Read the model definition and answer for the solid it produces. Units are mm, in the model's axes. Face numbers are marked on the shaded views. A direction names the side the tool comes from. Round coordinates to 2 decimals unless told otherwise and drop trailing zeros. Order: outer loops, then holes, each group sorted by start corner. A loop starts at its lowest first (then second) coordinate and runs counter-clockwise, first axis right, second up. Notation, with made-up numbers: (10.25, 32.25) - (17.25, 32.25) arc R8 ccw to (17.25, 37.25) - close; hole circle Ø7 at (-3, 83.25). An arc over 180 degrees is marked (long way). Answer as a JSON object with one key per item and string values. Group by question number.
Q1. The mould has two halves that part along Z. Classify the marked faces 1, 2, 3 and 4: pulls with the +Z half, pulls with the -Z half, needs draft (parallel to the pull), parting line crosses it, or undercut.
Q2. A tool of negligible diameter and unlimited length cuts with its end or side. For the marked faces 5, 6, 7 and 8, from which of +Z, -Z, +X, -X, +Y, -Y can it reach the whole face along a straight path? Write none if from no direction.
Q3. Consider line 1 (Z direction, x = 18.25, y = 0); line 2 (Z direction, x = 25.5, y = 13); line 3 (X direction, y = -1.5, z = 4.75). Determine where each line is inside the solid, lowest interval first.
Q4. A cutting plane is placed at D-D on z = 0. Determine the outline of the cut face in (x, y), and give its area (3 significant figures).
Q5. A cutting plane is placed at B-B on x = 16.75. Determine the outline of the cut face in (y, z), and give its area (3 significant figures).
Q6. A cutting plane is placed at C-C on y = 0. Determine the outline of the cut face in (x, z).
Q7. Given pin 1 Ø0.5 at (y, z) = (22, -4.5) entering from -X; pin 2 Ø1.1 at (y, z) = (23, -7) entering from +X; pin 3 Ø5 at (x, y) = (22, 23) entering from +Z; pin 4 Ø2.5 at (x, y) = (25, 12.5) entering from -Z, each flat-ended and moving along its own axis, determine where each tip first touches the part or whether it passes through.
Q8. A cutting plane is placed at A-A on y = 25. Determine the outline of the cut face in (x, z), and give its area (3 significant figures).
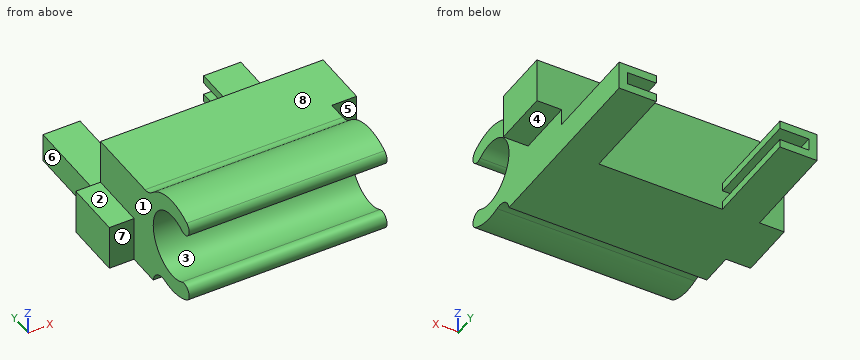
Autodesk Inventor part; units mm, degrees
ref_plane "YZ Plane" through (0, 0, 0) normal (1, 0, 0) x (0, 1, 0)
ref_plane "XZ Plane" through (0, 0, 0) normal (0, 1, 0) x (-1, 0, 0)
ref_plane "XY Plane" through (0, 0, 0) normal (0, 0, 1) x (1, 0, 0)
sketch "Sketch1" plane through (0, 0, 0) normal (1, 0, 0) x (0, 1, 0)
  circle A0 centre (0, 0) radius 4
  arc A1 (-3, -5.1962) -> (-3, 5.1962) centre (0, 0) ccw
  arc A2 (-3, 5.1962) -> (-2, 3.4641) centre (-2.5, 4.3301) ccw
  arc A3 (-2, -3.4641) -> (-3, -5.1962) centre (-2.5, -4.3301) ccw
  line L0 (15, 3.6) -> (4, 3.6)
  line L1 (4, 3.6) -> (4, -7.4)
  line L2 (4, -7.4) -> (15, -7.4)
  line L3 (15, -7.4) -> (15, 3.6)
  dimension "d0" = 8
  dimension "d1" = 12
  dimension "d2" = 2.5
  dimension "d4" = 11
  dimension "d5" = 11
  dimension "d6" = 4
  dimension "d9" = 7.4
extrude "Extrusion1" add sketch "Sketch1" along normal blind 24 contours L1 A1 A3 A0 | A0 A2 A1 L0 L1 | L1 L0 A1 | A1 L0 L3 L2 L1
fillet "Fillet1" radius 2 1 edges at (12, 4, -4.4721)
fillet "Fillet2" radius 2 1 edges at (12, 4.8, 3.6)
ref_plane "Work Plane1" through (0, 4.8, -6.4) normal (0, 0, 1) x (1, 0, 0)
sketch "Sketch5" plane through (24, 0, 0) normal (1, 0, 0) x (0, 0, -1)
  line L0 (-3.6, 15) -> (-3.6, 5.7131)
  line L1 (-3.6, 15) -> (1.9, 15)
  line L2 (1.9, 15) -> (1.9, 8)
  line L3 (1.9, 8) -> (-3.6, 8)
  line L4 (-3.6, 8) -> (-3.6, 15)
  point P0 (0, 0)
  dimension "d31" = 5.5
  dimension "d32" = 7
extrude "Extrusion5" add sketch "Sketch5" along normal blind 3
sketch "Sketch6" plane through (0, 0, 0) normal (-1, 0, 0) x (0, 0, 1)
  line L0 (-7.4, 4) -> (-7.4, 15)
  line L1 (-7.4, 15) -> (-1.9, 15)
  line L2 (-1.9, 15) -> (-1.9, 8)
  line L3 (-1.9, 8) -> (-7.4, 8)
  line L4 (-7.4, 8) -> (-7.4, 15)
  point P0 (0, 0)
  point P1 (-8, 4)
  dimension "d35" = 7
  dimension "d36" = 5.5
extrude "Extrusion6" add sketch "Sketch6" along normal blind 3
sketch "Sketch11" plane through (0, 15, 3.6) normal (0, 1, 0) x (1, 0, 0)
  line L0 (0, 11) -> (24, 11)
  line L1 (0, 5.5) -> (0, 11)
  line L2 (0, 11) -> (0, 7.5)
  line L3 (24, 7.5) -> (24, 11)
  line L4 (1, 8.5) -> (1, 10)
  line L5 (23, 10) -> (23, 8.5)
  line L6 (19.5, 8.5) -> (19.5, 7.5)
  line L7 (19.5, 10) -> (19.5, 11)
  line L8 (-3, 11) -> (24, 11)
  line L9 (4.5, 7.5) -> (4.5, 8.5)
  line L10 (4.5, 10) -> (4.5, 11)
  line L11 (19.5, 10) -> (19.5, 11)
  line L12 (18.3, 11) -> (21.5, 11)
  line L13 (1, 10) -> (4.5, 10)
  line L14 (19.5, 10) -> (23, 10)
  line L15 (24, 11) -> (19.5, 11)
  line L16 (4.5, 11) -> (0, 11)
  line L17 (23, 8.5) -> (19.5, 8.5)
  line L18 (4.5, 8.5) -> (1, 8.5)
  line L19 (0, 7.5) -> (4.5, 7.5)
  line L20 (19.5, 7.5) -> (24, 7.5)
  point P0 (0, 3.6)
  point P1 (23, 9.25)
  point P2 (24, 9.4038)
  point P3 (24, 9.25)
  point P4 (1, 9.25)
  point P5 (21.75, 7.5)
  point P6 (2.25, 7.5)
  point P7 (2.75, 8.5)
  point P8 (21.25, 8.5)
  point P9 (21.25, 10)
  point P10 (2.75, 10)
  point P11 (21.75, 11)
  point P12 (2.25, 11)
  dimension "d62" = 1.5
  dimension "d63" = 1
  dimension "d64" = 15
  dimension "d70" = 4.5
  dimension "d71" = 3.5
  dimension "d72" = 1
extrude "Extrusion10" add sketch "Sketch11" along normal blind 12
properties part number "Roller_Switch end"
Result set:
{
 "1": {"face 1": "needs draft", "face 2": "pulls with the +Z half", "face 3": "undercut", "face 4": "pulls with the -Z half"},
 "2": {"face 5": "+Z, -Z, +X, -Y", "face 6": "+Z, -Z, -X, +Y", "face 7": "+Z, -Z, -X, -Y", "face 8": "+Z, +X, -X, +Y"},
 "3": {"line 1": "z = -6 to -4, 4 to 6", "line 2": "z = -1.9 to 3.6", "line 3": "x = 0 to 24"},
 "4": {"outline": "(0, 4) - (24, 4) - (24, 8) - (27, 8) - (27, 15) - (0, 15) - close", "area": "285 mm²"},
 "5": {"outline": "(-3, -5.2) arc R6 ccw to (1.52, -5.8) arc R2 cw to (4, -7.4) - (15, -7.4) - (15, 3.6) - (5.71, 3.6) arc R2 cw to (4.28, 4.2) arc R6 ccw to (-3, 5.2) arc R1 ccw to (-2, 3.46) arc R4 cw (long way) to (-2, -3.46) arc R1 ccw to start", "area": "156 mm²"},
 "6": {"outline": "(0, -6) - (24, -6) - (24, -4) - (0, -4) - close; (0, 4) - (24, 4) - (24, 6) - (0, 6) - close"},
 "7": {"pin 1": "stops at x = 0", "pin 2": "stops at x = 24", "pin 3": "stops at z = -3.9", "pin 4": "stops at z = -7.4"},
 "8": {"outline": "(0, -7.4) - (4.5, -7.4) - (4.5, -6.4) - (1, -6.4) - (1, -4.9) - (4.5, -4.9) - (4.5, -3.9) - (0, -3.9) - close; (19.5, -7.4) - (24, -7.4) - (24, -3.9) - (19.5, -3.9) - (19.5, -4.9) - (23, -4.9) - (23, -6.4) - (19.5, -6.4) - close", "area": "21.0 mm²"}
}
